from build123d import *

# Parameters (mm, degrees)
F0_R     = 8.334375
F1_DEPTH = 2.38125
F2_R     = 6.746875
F3_DEPTH = 3.175
F4_SIZE  = 0.79375


with BuildPart() as f1:
    # F0 (on Top) → F1 (new body)
    with BuildSketch(Plane.XY):
        Circle(F0_R)
    extrude(amount=F1_DEPTH)

    # F2 (on face) → F3 (join)
    with BuildSketch(Plane.XY.offset(2.38125)):
        Circle(F2_R)
    extrude(amount=F3_DEPTH)

    # F4
    f4_edges = [f1.edges().sort_by_distance(p)[0] for p in [
        (-8.334375, 0, 2.38125),
        (-6.746875, 0, 5.55625),
    ]]
    chamfer(f4_edges, length=F4_SIZE)


solid = f1.part
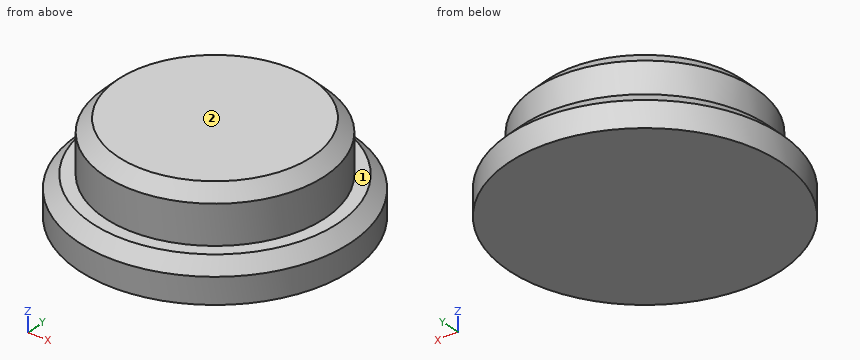
CAD build for the part. Positions are in the model's coordinates, mm. Face numbers are marked on the shaded views. A direction names the side the tool comes from. Round coordinates to 2 decimals unless told otherwise and drop trailing zeros. Write each loop counter-clockwise with the first axis right and the second up, starting at its lowest first coordinate (ties: lowest second). Pieces come first, ordered by that corner, then holes. Notation, with made-up numbers: M -8,-27 L 12,-27 A23 ccw 12,5 Z; hole C -5.5,-31 d2. An arc over 180 degrees is marked long. Use a Markdown table: item, result. Add a question column.
1. Flat gauge pins, fed straight in: P1, Ø1.5, axis at x = 5.5, y = 5, coming from the +Z side; P2, Ø2, axis at x = 3, z = 3, coming from the -Y side; P3, Ø1, axis at y = -4.5, z = 4.5, coming from the -X side. Where does each tip first touch, or does it go through?
2. Slice it at A-A on y = 0. Give the cut face in (x, z).
3. Slice it at D-D on z = 1.2. Give the cut face in (x, y), then the cut area to 3 significant figures.
4. Drill centre lines: probe 1 along Z at (x, y) = (1, -7.25); probe 2 along X at (y, z) = (-2.25, 2.5); probe 3 along X at (y, z) = (-1, 2.75). Where is each one in solid material? Low to high.
5. Slice it at C-C on z = 2.7. Give the cut face in (x, y).
6. 3-axis set-ups, long thin cutter, end or side, ignore diameter. For the marked faces 1 and 2: which of +Z, -Z, +X, -X, +Y, -Y reach the whole face in a straight line?
Reply:
| question | item | result |
|---|---|---|
| 1 | P1 | stops at z = 4.83 |
| 1 | P2 | stops at y = -7.4 |
| 1 | P3 | stops at x = -5.43 |
| 2 | outline | M -8.33,0 L 8.33,0 L 8.33,1.59 L 7.54,2.38 L 6.75,2.38 L 6.75,4.76 L 5.95,5.56 L -5.95,5.56 L -6.75,4.76 L -6.75,2.38 L -7.54,2.38 L -8.33,1.59 Z |
| 3 | outline | C 0,0 d16.67 |
| 3 | area | 218 mm^2 |
| 4 | probe 1 | z = 0 to 2.38 |
| 4 | probe 2 | x = -6.36 to 6.36 |
| 4 | probe 3 | x = -6.67 to 6.67 |
| 5 | outline | C 0,0 d13.49 |
| 6 | face 1 | +Z |
| 6 | face 2 | +Z, +X, -X, +Y, -Y |
